```python
from build123d import *

# Parameters (mm, degrees)
SKETCH_1_W                     = 3.125
SKETCH_1_H                     = 10.4
EXTRUDE_1_DEPTH                = 2.1
CUT_EXTRUDE_1_REACH            = 8.249
SKETCH_2_W                     = 6.25
SKETCH_2_H                     = 9
SKETCH_3_W                     = 1.55
SKETCH_3_H                     = 0.7
CUT_EXTRUDE_2_DEPTH            = 1.05
SKETCH_5_W                     = 1.55
SKETCH_5_H                     = 0.7
CUT_EXTRUDE_4_DEPTH            = 1.05
EXTRUDE_3_DEPTH                = 6.6
SKETCH_9_W                     = 2.8
SKETCH_9_H                     = 7.7
EXTRUDE_4_DEPTH                = 1.3
CUT_EXTRUDE_6_REACH            = 11.424
SKETCH_11_W                    = 1.8
SKETCH_11_H                    = 6.7
CUT_EXTRUDE_9_REACH            = 11.047
SKETCH_14_W                    = 1.8
SKETCH_14_H                    = 2.4
CUT_EXTRUDE_11_REACH           = 14.749
SKETCH_16_W                    = 1.55
SKETCH_16_H                    = 0.6
CUT_EXTRUDE_12_REACH           = 14.749
SKETCH_17_W                    = 1.55
SKETCH_17_H                    = 0.6
EXTRUDE_6_DEPTH                = 0.375
SKETCH_21_W                    = 0.8
SKETCH_21_H                    = 2.5
EXTRUDE_8_DEPTH                = 1.3
HOLE_WIZARD_2_1_2_1_2_D        = 2.1
HOLE_WIZARD_2_1_2_1_2_DEPTH    = 1.2
HOLE_WIZARD_1_2_1_2_1_D        = 1.2
FILLET_1_R                     = 0.4
PATTERN_LINEAR_1_COUNT         = 2
PATTERN_LINEAR_1_PITCH         = 3.5
FILLET_1_OF_PATTERN_LINEAR_1_R = 0.4


with BuildPart() as part:
    # Эскиз1 → Бобышка-Вытянуть1 (new body)
    with BuildSketch(Plane.XY.offset(1.05)):
        with Locations((-1.5625, 0)):
            Rectangle(SKETCH_1_W, SKETCH_1_H)
    extrude_1 = extrude(amount=-EXTRUDE_1_DEPTH)

    # Эскиз2 → Вырез-Вытянуть1 (cut, up to next)
    with BuildSketch(Plane(origin=(0, 0, -0.45), x_dir=(-1, 0, 0), z_dir=(0, 0, -1)), mode=Mode.PRIVATE) as cut_extrude_1_sk1:
        Rectangle(SKETCH_2_W, SKETCH_2_H)
    cut_extrude_1_tool1 = extrude(cut_extrude_1_sk1.sketch, amount=-CUT_EXTRUDE_1_REACH, mode=Mode.PRIVATE) & part.part
    cut_extrude_1 = cut_extrude_1_tool1.solids().sort_by_distance((0, 0, -0.45))[0]
    add(cut_extrude_1, mode=Mode.SUBTRACT)

    # Эскиз3 → Вырез-Вытянуть2 (cut)
    with BuildSketch(Plane(origin=(0, 0, -0.45), x_dir=(-1, 0, 0), z_dir=(0, 0, -1))):
        with Locations((1.75, 4.85)):
            Rectangle(SKETCH_3_W, SKETCH_3_H)
    cut_extrude_2 = extrude(amount=-CUT_EXTRUDE_2_DEPTH, mode=Mode.SUBTRACT)

    # Эскиз5 → Вырез-Вытянуть4 (cut)
    with BuildSketch(Plane(origin=(0, 0, -0.45), x_dir=(-1, 0, 0), z_dir=(0, 0, -1))):
        with Locations((1.75, -4.85)):
            Rectangle(SKETCH_5_W, SKETCH_5_H)
    cut_extrude_4 = extrude(amount=-CUT_EXTRUDE_4_DEPTH, mode=Mode.SUBTRACT)

    # Эскиз8 → Бобышка-Вытянуть3 (add)
    with BuildSketch(Plane(origin=(0, 0, -7.65), x_dir=(-1, 0, 0), z_dir=(0, 0, -1))):
        with BuildLine():
            Line((3.125, 2.05), (0.375, 2.05))
            Line((0.375, 2.05), (0.375, -2.05))
            ThreePointArc((0.375, -2.05), (1.75, -1.502368755), (3.125, -2.05))
            Line((3.125, -2.05), (3.125, 2.05))
        make_face()
    extrude_3 = extrude(amount=-EXTRUDE_3_DEPTH)

    # Эскиз9 → Бобышка-Вытянуть4 (add)
    with BuildSketch(Plane.XY.offset(0.85)):
        with Locations((-1.75, 0)):
            Rectangle(SKETCH_9_W, SKETCH_9_H)
    extrude_4 = extrude(amount=-EXTRUDE_4_DEPTH)

    # Эскиз11 → Вырез-Вытянуть6 (cut, up to next)
    with BuildSketch(Plane(origin=(0, 0, -0.45), x_dir=(-1, 0, 0), z_dir=(0, 0, -1)), mode=Mode.PRIVATE) as cut_extrude_6_sk1:
        with Locations((1.75, 0)):
            Rectangle(SKETCH_11_W, SKETCH_11_H)
    cut_extrude_6_tool1 = extrude(cut_extrude_6_sk1.sketch, amount=-CUT_EXTRUDE_6_REACH, mode=Mode.PRIVATE) & part.part
    cut_extrude_6 = cut_extrude_6_tool1.solids().sort_by_distance((-1.75, 0, -0.45))[0]
    add(cut_extrude_6, mode=Mode.SUBTRACT)

    # Эскиз14 → Вырез-Вытянуть9 (cut, up to next)
    with BuildSketch(Plane(origin=(0, 0, -5.65), x_dir=(-1, 0, 0), z_dir=(0, 0, -1)), mode=Mode.PRIVATE) as cut_extrude_9_sk1:
        with Locations((1.75, 0)):
            Rectangle(SKETCH_14_W, SKETCH_14_H)
    cut_extrude_9_tool1 = extrude(cut_extrude_9_sk1.sketch, amount=-CUT_EXTRUDE_9_REACH, mode=Mode.PRIVATE) & part.part
    cut_extrude_9 = cut_extrude_9_tool1.solids().sort_by_distance((-1.75, 0, -5.65))[0]
    add(cut_extrude_9, mode=Mode.SUBTRACT)

    # Эскиз16 → Вырез-Вытянуть11 (cut, up to next)
    with BuildSketch(Plane(origin=(0, -4.5, 0), x_dir=(1, 0, 0), z_dir=(0, 1, 0)), mode=Mode.PRIVATE) as cut_extrude_11_sk1:
        with Locations((-1.75, 0.75)):
            Rectangle(SKETCH_16_W, SKETCH_16_H)
    cut_extrude_11_tool1 = extrude(cut_extrude_11_sk1.sketch, amount=-CUT_EXTRUDE_11_REACH, mode=Mode.PRIVATE) & part.part
    cut_extrude_11 = cut_extrude_11_tool1.solids().sort_by_distance((-1.75, -4.5, -0.75))[0]
    add(cut_extrude_11, mode=Mode.SUBTRACT)

    # Эскиз17 → Вырез-Вытянуть12 (cut, up to next)
    with BuildSketch(Plane.XZ.offset(-4.5), mode=Mode.PRIVATE) as cut_extrude_12_sk1:
        with Locations((-1.75, -0.75)):
            Rectangle(SKETCH_17_W, SKETCH_17_H)
    cut_extrude_12_tool1 = extrude(cut_extrude_12_sk1.sketch, amount=-CUT_EXTRUDE_12_REACH, mode=Mode.PRIVATE) & part.part
    cut_extrude_12 = cut_extrude_12_tool1.solids().sort_by_distance((-1.75, 4.5, -0.75))[0]
    add(cut_extrude_12, mode=Mode.SUBTRACT)

    # Эскиз19 → Бобышка-Вытянуть6 (add)
    with BuildSketch(Plane(origin=(-3.5, 0, 0), x_dir=(0, -1, 0), z_dir=(-1, 0, 0))):
        Polygon((1.65, -1.05), (5.2, -1.05), (5.2, 1.046361901), (4.5, 1.046361901), (4.5, -0.453638099), (-4.5, -0.453638099), (-4.5, 1.046361901), (-5.2, 1.046361901), (-5.2, -1.05), align=None)
    extrude_6 = extrude(amount=-EXTRUDE_6_DEPTH)

    # Эскиз21 → Бобышка-Вытянуть8 (add)
    with BuildSketch(Plane(origin=(0, 3.35, 0), x_dir=(1, 0, 0), z_dir=(0, 1, 0))):
        with Locations((-1.75, 6.4)):
            Rectangle(SKETCH_21_W, SKETCH_21_H)
    extrude_8 = extrude(amount=-EXTRUDE_8_DEPTH)

    # Диаметр отверстия Ø2.1 (2.1)2
    with Locations(Plane(origin=(0, 0, -7.65), x_dir=(-1, 0, 0), z_dir=(0, 0, -1))):
        with Locations((1.75, 0)):
            hole_wizard_2_1_2_1_2 = Hole(HOLE_WIZARD_2_1_2_1_2_D / 2, depth=HOLE_WIZARD_2_1_2_1_2_DEPTH)

    # Диаметр отверстия Ø1.2 (1.2)1 (through all)
    with Locations(Plane.XY.offset(-5.65)):
        with Locations((-1.75, 0)):
            hole_wizard_1_2_1_2_1 = Hole(HOLE_WIZARD_1_2_1_2_1_D / 2)

    # Скругление1
    fillet_1_edges = [part.edges().sort_by_distance(p)[0] for p in [
        (-2.8, 0, -6.45),
    ]]
    fillet(fillet_1_edges, radius=FILLET_1_R)

    # Линейный массив1: Бобышка-Вытянуть1, Вырез-Вытянуть1, Вырез-Вытянуть2, Вырез-Вытянуть4, Бобышка-Вытянуть3, Бобышка-Вытянуть4, Вырез-Вытянуть6, Вырез-Вытянуть9, Вырез-Вытянуть11, Вырез-Вытянуть12, Бобышка-Вытянуть6, Бобышка-Вытянуть8, Диаметр отверстия Ø2.1 (2.1)2, Диаметр отверстия Ø1.2 (1.2)1 ×2
    with Locations(*[(-i * PATTERN_LINEAR_1_PITCH, 0, 0) for i in range(1, PATTERN_LINEAR_1_COUNT)]):
        add(extrude_1)
        add(cut_extrude_1, mode=Mode.SUBTRACT)
        add(cut_extrude_2, mode=Mode.SUBTRACT)
        add(cut_extrude_4, mode=Mode.SUBTRACT)
        add(extrude_3)
        add(extrude_4)
        add(cut_extrude_6, mode=Mode.SUBTRACT)
        add(cut_extrude_9, mode=Mode.SUBTRACT)
        add(cut_extrude_11, mode=Mode.SUBTRACT)
        add(cut_extrude_12, mode=Mode.SUBTRACT)
        add(extrude_6)
        add(extrude_8)
        add(hole_wizard_2_1_2_1_2, mode=Mode.SUBTRACT)
        add(hole_wizard_1_2_1_2_1, mode=Mode.SUBTRACT)

    # Скругление1 of Линейный массив1
    fillet_1_of_pattern_linear_1_edges = [part.edges().sort_by_distance(p)[0] for p in [
        (-6.3, 0, -6.45),
    ]]
    fillet(fillet_1_of_pattern_linear_1_edges, radius=FILLET_1_OF_PATTERN_LINEAR_1_R)


solid = part.part
```
Geometry check sheet. Reference: the model listing, model coordinates, mm. A direction names the side the tool comes from. Round coordinates to 2 decimals unless told otherwise and drop trailing zeros. Loops run counter-clockwise (first coordinate to the right, second up) from the corner with the lowest first, then second, coordinate; pieces in that order, holes last. Notation, with made-up numbers: M 81,81 L 90,81 A22 cw 90,105 Z; hole C 5.5,78 d3. An arc over 180 degrees is marked long. Return JSON: item names as keys, results as strings. Group by question number.
(1) Section check A-A, the plane z = -1.5. Enter the section's corners in (x, y) (3 decimals), and give its area (3 significant figures).
(2) Mould release check, pull along Z, two halves, no side actions. Record for faces 1 (the face through (-0.53, 0.05, 0.85)), 2 (the face through (-0.85, 0, -2)), 3 (the face through (-5, 2.05, -4)): pulls with the +Z half, pulls with the -Z half, needs draft (parallel to the pull), parting line crosses it, or undercut.
(3) Section check C-C, the plane x = -3. Enter the section's corners in (y, z).
(4) Set-up check for faces 4 (the face through (-5.229, -1.502, -4.396)), 5 (the face through (-2, -3.35, 0)), 6 (the face through (-0.375, 0, -4)), 7 (the face through (-4.03, 0.05, 0.85)): record each of +Z, -Z, +X, -X, +Y, -Y from which the full face is reachable in a straight line by a thin tool's end or side.
(5) Go/stop test with flat-tipped pins: pin 1 (0.6 mm diameter, centred on x = -5.5, y = -4.5, fed in from -Z); pin 2 (0.9 mm diameter, centred on x = -1.5, y = 3, fed in from +Z); pin 3 (1.4 mm diameter, centred on x = -2, z = 0, fed in from +Y); pin 4 (0.7 mm diameter, centred on x = -5, z = -0.5, fed in from +Y). Record where each tip stops, or that it passes through.
(6) Scan lines: line 1 along X through (y, z) = (0, -4.5) (3 decimals); line 2 along X through (y, z) = (4.75, -0.75) (3 decimals); line 3 along Z through (x, y) = (-5, 2.5). Record each from-to range of solid material in increasing order. Write a range as [from, to].
(7) Section check B-B, the plane y = 2.5. Give the number of separate pieces and of enclosed holes in the cut face, and give its area (3 significant figures).
Data:
{
 "1": {"outline": "M -6.625,-2.05 A2 cw -3.875,-2.05 L -3.875,2.05 L -6.625,2.05 Z; M -3.125,-2.05 A2 cw -0.375,-2.05 L -0.375,2.05 L -3.125,2.05 Z; hole M -6.15,-1.2 L -4.35,-1.2 L -4.35,1.2 L -6.15,1.2 Z; hole M -2.65,-1.2 L -0.85,-1.2 L -0.85,1.2 L -2.65,1.2 Z", "area": "11.8 mm²"},
 "2": {"face 1": "pulls with the +Z half", "face 2": "needs draft", "face 3": "undercut"},
 "3": {"outline": "M -5.2,-1.05 L -1.94,-1.05 L -1.94,-7.65 L 2.05,-7.65 L 2.05,-1.05 L 5.2,-1.05 L 5.2,1.05 L 4.5,1.05 L 4.5,-0.45 L 3.85,-0.45 L 3.85,0.85 L -3.85,0.85 L -3.85,-0.45 L -4.5,-0.45 L -4.5,1.05 L -5.2,1.05 Z"},
 "4": {"face 4": "-Z, -Y", "face 5": "+Z", "face 6": "-Z, +X, +Y, -Y", "face 7": "+Z, +X, -X"},
 "5": {"pin 1": "z = -1.05", "pin 2": "z = 0.85", "pin 3": "y = 5.2", "pin 4": "y = 4.5"},
 "6": {"line 1": "[-6.625, -6.15], [-4.35, -3.875], [-3.125, -2.65], [-0.85, -0.375]", "line 2": "[-7, -6.025], [-4.475, -2.525], [-0.975, 0]", "line 3": "[-7.65, -5.15], [-1.05, -0.45]"},
 "7": {"separate pieces": "3", "enclosed holes": "0", "area": "10.8 mm²"}
}
